```python
from build123d import *

# Parameters (mm, degrees)
F1_DEPTH = 25
F2_DEPTH = 8
F3_DEPTH = 25
F4_DEPTH = 15
F6_DEPTH = 15
F7_D     = 4
F8_R     = 5


with BuildPart() as f1:
    # F0 (on Front) → F1 (new body)
    with BuildSketch(Plane.XZ):
        with BuildLine():
            Line((-349.5359115523, -100.9652705431), (-336.307154997, -85.9652705431))
            ThreePointArc((-336.307154997, -85.9652705431), (-353.178144257, -76.1627254717), (-372.5163375921, -73.5637935721))
            ThreePointArc((-372.5163375921, -73.5637935721), (-390.430756518, -78.1130324452), (-405.4684846867, -88.8595998648))
            ThreePointArc((-405.4684846867, -88.8595998648), (-413.3268873379, -147.310338704), (-360.0407755432, -172.5854975141))
            ThreePointArc((-360.0407755432, -172.5854975141), (-343.7235260202, -166.3814012494), (-330.5336171349, -154.9459412214))
            ThreePointArc((-330.5336171349, -154.9459412214), (-322.250119692, -140.1645001283), (-319.3790463853, -123.4652705431))
            ThreePointArc((-319.3790463853, -123.4652705431), (-319.4771834235, -120.3341249159), (-319.7712093028, -117.2152705431))
            Line((-319.7712093028, -117.2152705431), (-339.6143441358, -119.7152705431))
            ThreePointArc((-339.6143441358, -119.7152705431), (-339.4379286082, -121.5865831668), (-339.3790463853, -123.4652705431))
            ThreePointArc((-339.3790463853, -123.4652705431), (-396.7221812183, -135.8084053761), (-349.5359115523, -100.9652705431))
        make_face()
        with BuildLine():
            ThreePointArc((-319.7712093028, -117.2152705431), (-325.1848725611, -100.0799118758), (-336.307154997, -85.9652705431))
            Line((-336.307154997, -85.9652705431), (-349.5359115523, -100.9652705431))
            ThreePointArc((-349.5359115523, -100.9652705431), (-342.8625420908, -109.4340553427), (-339.6143441358, -119.7152705431))
            Line((-339.6143441358, -119.7152705431), (-319.7712093028, -117.2152705431))
        make_face()
        with BuildLine():
            Line((-336.307154997, -85.9652705431), (-322.6025679954, -70.4257295315))
            Line((-322.6025679954, -70.4257295315), (-372.5163375921, -73.5637935721))
            ThreePointArc((-372.5163375921, -73.5637935721), (-353.178144257, -76.1627254717), (-336.307154997, -85.9652705431))
        make_face()
        with BuildLine():
            Line((-322.6025679954, -70.4257295315), (10.9477045802, 307.7847294569))
            ThreePointArc((10.9477045802, 307.7847294569), (2.5055132487, 325.4894205434), (9.4389311237, 343.837564796))
            Line((9.4389311237, 343.837564796), (-405.4684846867, -88.8595998648))
            ThreePointArc((-405.4684846867, -88.8595998648), (-390.430756518, -78.1130324452), (-372.5163375921, -73.5637935721))
            Line((-372.5163375921, -73.5637935721), (-322.6025679954, -70.4257295315))
        make_face()
        with BuildLine():
            ThreePointArc((27.4836502744, 301.5347294569), (18.6448155096, 303.1493707896), (10.9477045802, 307.7847294569))
            Line((10.9477045802, 307.7847294569), (-322.6025679954, -70.4257295315))
            Line((-322.6025679954, -70.4257295315), (-258.7862584205, -66.4136168841))
            Line((-258.7862584205, -66.4136168841), (-79.1806184856, 155.209939055))
            Line((-79.1806184856, 155.209939055), (27.4836502744, 286.8278244556))
            Line((27.4836502744, 286.8278244556), (27.4836502744, 301.5347294569))
        make_face()
        with BuildLine():
            Line((-258.7862584205, -66.4136168841), (-322.6025679954, -70.4257295315))
            Line((-322.6025679954, -70.4257295315), (-336.307154997, -85.9652705431))
            ThreePointArc((-336.307154997, -85.9652705431), (-325.1848725611, -100.0799118758), (-319.7712093028, -117.2152705431))
            Line((-319.7712093028, -117.2152705431), (-297.7031676779, -114.4349586354))
            Line((-297.7031676779, -114.4349586354), (-258.7862584205, -66.4136168841))
        make_face()
        with BuildLine():
            Line((-79.1806184856, 155.209939055), (-258.7862584205, -66.4136168841))
            Line((-258.7862584205, -66.4136168841), (25.915004671, -48.5145320576))
            ThreePointArc((25.915004671, -48.5145320576), (-93.174775765, 19.0206064889), (-79.1806184856, 155.209939055))
        make_face()
        with BuildLine():
            Line((13.8414950767, -75.1840205431), (2.6797317332, -76.5902705431))
            ThreePointArc((2.6797317332, -76.5902705431), (12.7792837339, -93.6836187606), (32.1527856955, -98.0253840286))
            ThreePointArc((32.1527856955, -98.0253840286), (46.7414848558, -89.4069080762), (52.4836502744, -73.4652705431))
            ThreePointArc((52.4836502744, -73.4652705431), (45.1613198041, -55.7876010134), (27.4836502744, -48.4652705431))
            Line((27.4836502744, -48.4652705431), (27.4836502744, -59.7152705431))
            ThreePointArc((27.4836502744, -59.7152705431), (37.2063685157, -63.7425523018), (41.2336502744, -73.4652705431))
            ThreePointArc((41.2336502744, -73.4652705431), (28.3447153219, -87.1882828576), (13.8414950767, -75.1840205431))
        make_face()
        with BuildLine():
            Line((2.6797317332, -76.5902705431), (-297.7031676779, -114.4349586354))
            Line((-297.7031676779, -114.4349586354), (-330.5336171349, -154.9459412214))
            ThreePointArc((-330.5336171349, -154.9459412214), (-343.7235260202, -166.3814012494), (-360.0407755432, -172.5854975141))
            Line((-360.0407755432, -172.5854975141), (32.1527856955, -98.0253840286))
            ThreePointArc((32.1527856955, -98.0253840286), (12.7792837339, -93.6836187606), (2.6797317332, -76.5902705431))
        make_face()
        with BuildLine():
            ThreePointArc((27.4836502744, -48.4652705431), (26.6989408177, -48.4775889566), (25.915004671, -48.5145320576))
            ThreePointArc((25.915004671, -48.5145320576), (8.223852566, -57.5260048062), (2.6797317332, -76.5902705431))
            Line((2.6797317332, -76.5902705431), (13.8414950767, -75.1840205431))
            ThreePointArc((13.8414950767, -75.1840205431), (17.1711502744, -64.3705004113), (27.4836502744, -59.7152705431))
            Line((27.4836502744, -59.7152705431), (27.4836502744, -48.4652705431))
        make_face()
        with BuildLine():
            Line((25.915004671, -48.5145320576), (-258.7862584205, -66.4136168841))
            Line((-258.7862584205, -66.4136168841), (-297.7031676779, -114.4349586354))
            Line((-297.7031676779, -114.4349586354), (2.6797317332, -76.5902705431))
            ThreePointArc((2.6797317332, -76.5902705431), (8.223852566, -57.5260048062), (25.915004671, -48.5145320576))
        make_face()
        with BuildLine():
            Line((-297.7031676779, -114.4349586354), (-319.7712093028, -117.2152705431))
            ThreePointArc((-319.7712093028, -117.2152705431), (-319.4771834235, -120.3341249159), (-319.3790463853, -123.4652705431))
            ThreePointArc((-319.3790463853, -123.4652705431), (-322.250119692, -140.1645001283), (-330.5336171349, -154.9459412214))
            Line((-330.5336171349, -154.9459412214), (-297.7031676779, -114.4349586354))
        make_face()
        with BuildLine():
            ThreePointArc((46.9063648996, 310.7943941178), (38.2421728617, 303.9680683893), (27.4836502744, 301.5347294569))
            Line((27.4836502744, 301.5347294569), (27.4836502744, 286.8278244556))
            Line((27.4836502744, 286.8278244556), (46.9063648996, 310.7943941178))
        make_face()
        with BuildLine():
            Line((10.9477045802, 307.7847294569), (18.3888801426, 316.2222294569))
            ThreePointArc((18.3888801426, 316.2222294569), (21.8263801426, 339.0669995887), (41.2336502744, 326.5347294569))
            ThreePointArc((41.2336502744, 326.5347294569), (37.2063685157, 316.8120112156), (27.4836502744, 312.7847294569))
            Line((27.4836502744, 312.7847294569), (27.4836502744, 301.5347294569))
            ThreePointArc((27.4836502744, 301.5347294569), (38.2421728617, 303.9680683893), (46.9063648996, 310.7943941178))
            ThreePointArc((46.9063648996, 310.7943941178), (51.048113621, 318.1851146643), (52.4836502744, 326.5347294569))
            ThreePointArc((52.4836502744, 326.5347294569), (36.8078666284, 349.730828038), (9.4389311237, 343.837564796))
            ThreePointArc((9.4389311237, 343.837564796), (2.5055132487, 325.4894205434), (10.9477045802, 307.7847294569))
        make_face()
        with BuildLine():
            ThreePointArc((27.4836502744, 312.7847294569), (22.6222911537, 313.6727821899), (18.3888801426, 316.2222294569))
            Line((18.3888801426, 316.2222294569), (10.9477045802, 307.7847294569))
            ThreePointArc((10.9477045802, 307.7847294569), (18.6448155096, 303.1493707896), (27.4836502744, 301.5347294569))
            Line((27.4836502744, 301.5347294569), (27.4836502744, 312.7847294569))
        make_face()
    extrude(amount=F1_DEPTH)

    # F0 (on Front) → F2 (join)
    with BuildSketch(Plane.XZ):
        with BuildLine():
            ThreePointArc((27.4836502744, -59.7152705431), (17.1711502744, -64.3705004113), (13.8414950767, -75.1840205431))
            Line((13.8414950767, -75.1840205431), (27.4836502744, -73.4652705431))
            Line((27.4836502744, -73.4652705431), (27.4836502744, -59.7152705431))
        make_face()
        with BuildLine():
            Line((27.4836502744, -73.4652705431), (13.8414950767, -75.1840205431))
            ThreePointArc((13.8414950767, -75.1840205431), (28.3447153219, -87.1882828576), (41.2336502744, -73.4652705431))
            ThreePointArc((41.2336502744, -73.4652705431), (37.2063685157, -63.7425523018), (27.4836502744, -59.7152705431))
            Line((27.4836502744, -59.7152705431), (27.4836502744, -73.4652705431))
        make_face()
        with BuildLine():
            Line((27.4836502744, 312.7847294569), (27.4836502744, 326.5347294569))
            Line((27.4836502744, 326.5347294569), (18.3888801426, 316.2222294569))
            ThreePointArc((18.3888801426, 316.2222294569), (22.6222911537, 313.6727821899), (27.4836502744, 312.7847294569))
        make_face()
        with BuildLine():
            Line((18.3888801426, 316.2222294569), (27.4836502744, 326.5347294569))
            Line((27.4836502744, 326.5347294569), (27.4836502744, 312.7847294569))
            ThreePointArc((27.4836502744, 312.7847294569), (37.2063685157, 316.8120112156), (41.2336502744, 326.5347294569))
            ThreePointArc((41.2336502744, 326.5347294569), (21.8263801426, 339.0669995887), (18.3888801426, 316.2222294569))
        make_face()
    extrude(amount=F2_DEPTH)

    # F0 (on Front) → F3 (join)
    with BuildSketch(Plane.XZ):
        with BuildLine():
            Line((-369.3790463853, -123.4652705431), (-349.5359115523, -100.9652705431))
            ThreePointArc((-349.5359115523, -100.9652705431), (-396.7221812183, -135.8084053761), (-339.3790463853, -123.4652705431))
            ThreePointArc((-339.3790463853, -123.4652705431), (-339.4379286082, -121.5865831668), (-339.6143441358, -119.7152705431))
            Line((-339.6143441358, -119.7152705431), (-369.3790463853, -123.4652705431))
        make_face()
        with BuildLine():
            ThreePointArc((-339.6143441358, -119.7152705431), (-342.8625420908, -109.4340553427), (-349.5359115523, -100.9652705431))
            Line((-349.5359115523, -100.9652705431), (-369.3790463853, -123.4652705431))
            Line((-369.3790463853, -123.4652705431), (-339.6143441358, -119.7152705431))
        make_face()
    extrude(amount=F3_DEPTH)

    # F0 (on Front) → F4 (cut)
    with BuildSketch(Plane.XZ):
        with BuildLine():
            ThreePointArc((-339.6143441358, -119.7152705431), (-342.8625420908, -109.4340553427), (-349.5359115523, -100.9652705431))
            Line((-349.5359115523, -100.9652705431), (-369.3790463853, -123.4652705431))
            Line((-369.3790463853, -123.4652705431), (-339.6143441358, -119.7152705431))
        make_face()
        with BuildLine():
            Line((-369.3790463853, -123.4652705431), (-349.5359115523, -100.9652705431))
            ThreePointArc((-349.5359115523, -100.9652705431), (-396.7221812183, -135.8084053761), (-339.3790463853, -123.4652705431))
            ThreePointArc((-339.3790463853, -123.4652705431), (-339.4379286082, -121.5865831668), (-339.6143441358, -119.7152705431))
            Line((-339.6143441358, -119.7152705431), (-369.3790463853, -123.4652705431))
        make_face()
    extrude(amount=F4_DEPTH, mode=Mode.SUBTRACT)

    # F5 (on Front) → F6 (cut)
    with BuildSketch(Plane.XZ):
        Polygon((-369.3790463853, -123.4652705431), (-368.7540463853, -128.4260542513), (28.1086502744, -78.4260542513), (26.8586502744, -68.5044868349), (-356.8790463853, -116.8508922654), (-365.6290463853, -126.7724596819), align=None)
        Polygon((-373.1290463853, -120.1580814043), (-369.3790463853, -123.4652705431), (-370.0040463853, -118.5044868349), (-356.8790463853, -116.8508922654), (31.2336502744, 323.2275403181), (23.7336502744, 329.8419185957), align=None)
    extrude(amount=F6_DEPTH, mode=Mode.SUBTRACT)

    # F7 (through all)
    with Locations(Plane(origin=(0, 0, 0), x_dir=(1, 0, 0), z_dir=(0, 1, 0))):
        with Locations((-369.3790463853, 123.4652705431)):
            Hole(F7_D / 2)

    # F8
    f8_edges = [f1.edges().sort_by_distance(p)[0] for p in [
        (-198.014777, -25, 127.488982),
    ]]
    fillet(f8_edges, radius=F8_R)


solid = f1.part
```
Part model, mm, in its own coordinate system. A direction names the side the tool comes from. Give positions to 0.01 mm unless a question says otherwise; leave off trailing zeros. Return JSON: item names as keys, results as strings.
1) Pull direction Y, two halves, no side cores. Call faces 6 (the face through (-92.23, -9.86, 17.226)), 7 (the face through (-185, -25, -5)), 8 (the face through (-167, 0, 12)): released by +Y, released by -Y, zero draft, split by the parting line, or undercut.
Calculated:
{"face 6": "zero draft", "face 7": "released by -Y", "face 8": "released by +Y"}
2) Flat gauge pins, fed straight in: pin 1 Ø10 at (x, y) = (-327, -13) entering from +Z; pin 2 Ø10 at (x, y) = (-18.5, -18.5) entering from +Z; pin 3 Ø2 at (x, y) = (-340, -6) entering from -Z. Where does each tip first touch, or does it go through?
Calculated:
{"pin 1": "stops at z = -1.81", "pin 2": "stops at z = 319.92", "pin 3": "stops at z = -168.97"}
3) 3-axis set-ups, long thin cutter, end or side, ignore diameter. For faces 1 (the face through (30, -8, 327)), 2 (the face through (-16.362, -23.496, 234.989)), 3 (the face through (-199.89, -23.5, 123.47)), 4 (the face through (-158.2, -7.4, -101.9)), 5 (the face through (-17.02, -9.86, 231.91)): which of +Z, -Z, +X, -X, +Y, -Y reach the whole face in a straight line?
Calculated:
{"face 1": "-Y", "face 2": "+X, -Y", "face 3": "+Z, -X, -Y", "face 4": "+Y", "face 5": "+X, +Y, -Y"}
4) Drill centre lines: line 1 (Z direction, x = 13, y = -9.25); line 2 (Z direction, x = -83, y = -12.75); line 3 (Z direction, x = -245, y = -14.25). Where is each one in solid material? Low to high.
Calculated:
{"line 1": "z = -101.67 to -80.33, -70.25 to -48.66, 268.96 to 302.55, 317.67 to 346.91", "line 2": "z = -119.92 to -92.42, -82.35 to 2.56, 150.25 to 193.7, 208.82 to 247.44", "line 3": "z = -150.72 to -112.83, -102.76 to 10.01, 25.13 to 78.49"}
